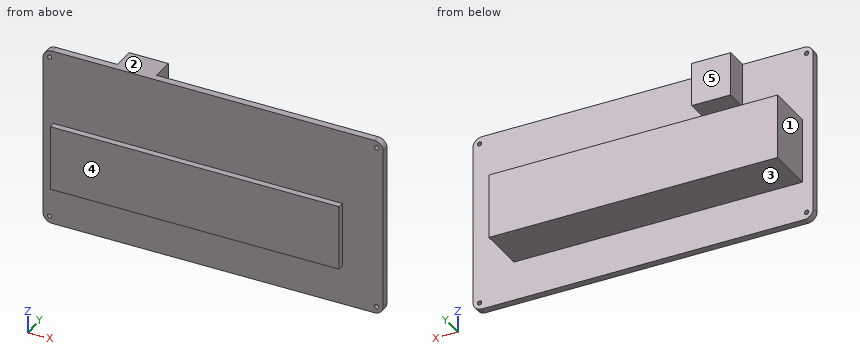
```python
from build123d import *

# Parameters (mm, degrees)
ESQUISSE1_W                                = 76
ESQUISSE1_H                                = 40
BOSS_EXTRU_1_DEPTH                         = 1.6
CONG_1_R                                   = 2
ESQUISSE2_R                                = 0.479748543
ENL_V_MAT_EXTRU_1_DEPTH                    = 1.6
SYM_TRIE1_AT_THE_SECOND_PLANE_COPY_1_SKE_R = 0.479748543
SYM_TRIE1_AT_THE_SECOND_PLANE_COPY_1_DEPTH = 1.6
BOSS_EXTRU_2_DEPTH                         = 10.5
BOSS_EXTRU_2_DEPTH_BACK                    = 3
ESQUISSE3_W                                = 64.5
ESQUISSE3_H                                = 14.5
ESQUISSE4_W                                = 8.707519808
ESQUISSE4_H                                = 9.784752996
BOSS_EXTRU_3_DEPTH                         = 5


with BuildPart() as part:
    # Esquisse1 → Boss.-Extru.1 (new body)
    with BuildSketch(Plane(origin=(0, 0, 0), x_dir=(1, 0, 0), z_dir=(0, 1, 0))):
        Rectangle(ESQUISSE1_W, ESQUISSE1_H)
    extrude(amount=BOSS_EXTRU_1_DEPTH)

    # Congé1
    cong_1_edges = [part.edges().sort_by_distance(p)[0] for p in [
        (38, 0.8, 20),
        (-38, 0.8, 20),
        (-38, 0.8, -20),
        (38, 0.8, -20),
    ]]
    fillet(cong_1_edges, radius=CONG_1_R)

    # Esquisse2 → Enlèv. mat.-Extru.1 (cut)
    with BuildSketch(Plane(origin=(0, 1.6, 0), x_dir=(1, 0, 0), z_dir=(0, 1, 0))):
        with Locations(Location((-36.533901181, -18.459426324, 0), (0, 0, 270))):
            Circle(ESQUISSE2_R)
    enl_v_mat_extru_1 = extrude(amount=-ENL_V_MAT_EXTRU_1_DEPTH, mode=Mode.SUBTRACT)

    # Symétrie1: Enlèv. mat.-Extru.1 across plane
    add(enl_v_mat_extru_1.mirror(Plane(origin=(0, 0, 0), x_dir=(0, 0, 1), z_dir=(1, 0, 0))), mode=Mode.SUBTRACT)

    # Symétrie1 at the second plane: Enlèv. mat.-Extru.1 across plane
    add(enl_v_mat_extru_1.mirror(Plane.XY), mode=Mode.SUBTRACT)

    # Symétrie1 at the second plane copy 1 ske → Symétrie1 at the second plane copy 1 (cut)
    with BuildSketch(Plane(origin=(0, 1.6, 0), x_dir=(-1, 0, 0), z_dir=(0, 1, 0))):
        with Locations(Location((-36.533901181, -18.459426324, 0), (0, 0, 270))):
            Circle(SYM_TRIE1_AT_THE_SECOND_PLANE_COPY_1_SKE_R)
    extrude(amount=-SYM_TRIE1_AT_THE_SECOND_PLANE_COPY_1_DEPTH, mode=Mode.SUBTRACT)

    # Esquisse3 → Boss.-Extru.2 (add, two sides: drawn at the far end of the back side and taken through both)
    with BuildSketch(Plane(origin=(0, 1.6, 0), x_dir=(1, 0, 0), z_dir=(0, 1, 0)).offset(-BOSS_EXTRU_2_DEPTH_BACK)):
        with Locations((-3.35, 3.932898171)):
            Rectangle(ESQUISSE3_W, ESQUISSE3_H)
    extrude(amount=BOSS_EXTRU_2_DEPTH + BOSS_EXTRU_2_DEPTH_BACK)

    # Esquisse4 → Boss.-Extru.3 (add)
    with BuildSketch(Plane(origin=(0, 1.6, 0), x_dir=(1, 0, 0), z_dir=(0, 1, 0))):
        with Locations((-17.853759904, -15.107623502)):
            Rectangle(ESQUISSE4_W, ESQUISSE4_H)
    extrude(amount=BOSS_EXTRU_3_DEPTH)


solid = part.part
```
Work out the finished part from the listing and answer in its coordinate system (mm). Face numbers are marked on the shaded views. A direction names the side the tool comes from. Give positions to 0.01 mm unless a question says otherwise; leave off trailing zeros. Order: outer loops, then holes, each group sorted by start corner. A loop starts at its lowest first (then second) coordinate and runs counter-clockwise, first axis right, second up. Notation, with made-up numbers: M -6,-5 L 19,-5 A13 ccw 19,12 Z; hole C 37,-14.75 d6. An arc over 180 degrees is marked long. Return JSON: item names as keys, results as strings.
1) A tool of negligible diameter and unlimited length cuts with its end or side. For the marked faces 4 and 5, from which of +Z, -Z, +X, -X, +Y, -Y can it reach the whole face along a straight path? Write none if from no direction.
Resolved:
{"face 4": "+Z, -Z, +X, -X, -Y", "face 5": "+Z, +X, -X, +Y"}
2) Section B-B, the plane y = 2.5 is taken. Write down the section's boundary in (x, z).
Resolved:
{"outline": "M -35.6,-11.18 L 28.9,-11.18 L 28.9,3.32 L -35.6,3.32 Z; M -22.21,10.22 L -13.5,10.22 L -13.5,20 L -22.21,20 Z"}
3) For a pull along Z with two mould halves and no side action, classify the marked faces 1, 2 and 3 as +Z half, -Z half, draft (parallel to the pull), parting line (faces both ways), or undercut.
Resolved:
{"face 1": "draft", "face 2": "+Z half", "face 3": "-Z half"}
4) Section D-D, the plane y = 9.75 is taken. Write down the section's boundary in (x, z), plus the area to 3 significant figures.
Resolved:
{"outline": "M -35.6,-11.18 L 28.9,-11.18 L 28.9,3.32 L -35.6,3.32 Z", "area": "935 mm^2"}
5) Section C-C, the plane x = -7 is taken. Write down the section's boundary in (y, z), plus the area to 3 significant figures.
Resolved:
{"outline": "M -1.4,-11.18 L 0,-11.18 L 0,-20 L 1.6,-20 L 1.6,-11.18 L 12.1,-11.18 L 12.1,3.32 L 1.6,3.32 L 1.6,20 L 0,20 L 0,3.32 L -1.4,3.32 Z", "area": "237 mm^2"}
6) Section A-A, the plane z = -7 is taken. Write down the section's boundary in (x, y).
Resolved:
{"outline": "M -38,0 L -35.6,0 L -35.6,-1.4 L 28.9,-1.4 L 28.9,0 L 38,0 L 38,1.6 L 28.9,1.6 L 28.9,12.1 L -35.6,12.1 L -35.6,1.6 L -38,1.6 Z"}
7) Each of these flat-tipped pins is pushed along its axis until it touches: pin 1 (3 mm diameter, centred on x = 3, y = 6, fed in from -Z); pin 2 (5 mm diameter, centred on y = 10, z = -7.5, fed in from +X); pin 3 (9.5 mm diameter, centred on x = -19, z = 16, fed in from +Y); pin 4 (1.5 mm diameter, centred on y = -0.5, z = -3, fed in from -X). Where does it stop, or does it pass through?
Resolved:
{"pin 1": "z = -11.18", "pin 2": "x = 28.9", "pin 3": "y = 6.6", "pin 4": "x = -38"}
8) Straight lines are drawn through the part: line 1 along Z through (x, y) = (-18.5, 5.5); line 2 along Z through (x, y) = (-8.5, 3.75); line 3 along X through (y, z) = (5.5, 2). For each, find the intervals that lie inside material, in ascending order. Write a range as [from, to].
Resolved:
{"line 1": "[-11.18, 3.32], [10.22, 20]", "line 2": "[-11.18, 3.32]", "line 3": "[-35.6, 28.9]"}
